For this review, take the finished solid that the model builds, in its own axes (mm). A direction names the side the tool comes from. Coordinates: 2 decimals unless noted, no trailing zeros. Write each loop counter-clockwise with the first axis right and the second up, starting at its lowest first coordinate (ties: lowest second). Pieces come first, ordered by that corner, then holes.
1) We need section D-D on y = 15.8. Write out the cut boundary in (x, z).
2) For faces 4 (the face through (28, 16, 0)), 5 (the face through (36, -35.8, -48)), 6 (the face through (26, 12, 0)), list the 3-axis set-ups (+Z, -Z, +X, -X, +Y, -Y) from which the entire face can be reached by the end or side of a thin tool; tool diameter is ignored.
3) We need section A-A on x = 30. Write out the cut boundary in (y, z).
4) To check wall thickness, follow line 1 along Y through (x, z) = (22, 0); line 2 along X through (y, z) = (-30.75, -64); line 3 along Y through (x, z) = (23.5, 0.5). State the ranges of each line that lie inside material, in increasing order.
5) Mouldability with a two-part tool opening along Y and no side actions: class faces 1 (the face through (34, -12, 28)), 2 (the face through (28.1, -39.7, -0.4)), 3 (the face through (36, -19.8, -48)) as pulls with the +Y half, pulls with the -Y half, needs draft (parallel to the pull), parting line crosses it, or undercut.
6) Insertion check: P1, Ø4.5, axis at y = -24.2, z = -16, coming from the -X side; P2, Ø8, axis at x = 31, z = -39.5, coming from the -Y side; P3, Ø2, axis at y = -33, z = -56.5, coming from the -X side. Each pin has a flat end and moves straight along its axis. Give the tip position at first contact, or say it passes through.
Autodesk Inventor part; units mm, degrees
ref_plane "YZ Plane" through (0, 0, 0) normal (1, 0, 0) x (0, 1, 0)
ref_plane "XZ Plane" through (0, 0, 0) normal (0, 1, 0) x (-1, 0, 0)
ref_plane "XY Plane" through (0, 0, 0) normal (0, 0, 1) x (1, 0, 0)
sketch "Sketch1" plane through (0, 0, 0) normal (1, 0, 0) x (0, 1, 0)
  line L0 (-19.8, 28) -> (19.8, 28)
  line L1 (19.8, 28) -> (19.8, -28)
  line L2 (19.8, -28) -> (-19.8, -28)
  line L3 (-19.8, -28) -> (-19.8, 28)
  line L4 (-19.8, 28) -> (19.8, -28) construction
  line L5 (19.8, 28) -> (-19.8, -28) construction
  point P0 (0, 0)
  dimension "d0" = 39.6
  dimension "d1" = 56
extrude "Extrusion1" add sketch "Sketch1" along normal blind 40
sketch "Sketch2" plane through (0, -19.8, 28) normal (0, 0, 1) x (1, 0, 0)
  line L0 (7.8, 0) -> (32.2, 0)
  line L1 (32.2, 0) -> (32.2, 31.8)
  line L2 (32.2, 31.8) -> (7.8, 31.8)
  line L3 (7.8, 31.8) -> (7.8, 0)
  line L4 (0, 0) -> (40, 0)
  line L5 (40, 39.6) -> (40, 0)
  dimension "d4" = 24.4
  dimension "d5" = 31.8
  dimension "d6" = 7.8
extrude "Extrusion2" cut sketch "Sketch2" against normal blind 64
sketch "Sketch3" plane through (32.2, -19.8, 28) normal (-1, 0, 0) x (0, 0, 1)
  circle A0 centre (-12, 3.8502) radius 2.3
  circle A1 centre (-28, 3.8502) radius 2.3
  line L0 (0, 31.8) -> (0, 0)
  point P0 (-28, 19.8)
  dimension "d9" = 4.6
  dimension "d10" = 4.6
  dimension "d11" = 16
  dimension "d12" = 12
extrude "Extrusion3" add sketch "Sketch3" along normal blind 26
sketch "Sketch4" plane through (7.8, -19.8, 28) normal (1, 0, 0) x (0, 0, -1)
  line L0 (56, 0) -> (0, 0)
  line L1 (56, 0) -> (32, 0)
  line L2 (32, 0) -> (32, 8)
  line L3 (32, 8) -> (56, 8)
  line L4 (56, 8) -> (56, 0)
  point P0 (28, 19.8)
  point P1 (32, 0)
  dimension "d15" = 24
  dimension "d16" = 8
extrude "Extrusion4" add sketch "Sketch4" along normal blind 26
sketch "Sketch14" plane through (0, 19.8, 28) normal (0, 1, 0) x (1, 0, 0)
  line L0 (20, 0) -> (20, 56)
  point P0 (0, 28)
sketch "Sketch15" plane through (0, -19.8, -28) normal (0, -1, 0) x (1, 0, 0)
  line L0 (40, 0) -> (40, 56)
  line L1 (0, 0) -> (40, 0)
  line L2 (0, 56) -> (40, 56)
  line L3 (0, 0) -> (0, 56)
  point P0 (0, 28)
extrude "Extrusion7" add sketch "Sketch15" along normal blind 24
sketch "Sketch16" plane through (0, 19.8, 28) normal (0, 0, 1) x (1, 0, 0)
  line L0 (8, -47.6) -> (32, -47.6)
  line L1 (32, -47.6) -> (32, -55.6)
  line L2 (32, -55.6) -> (8, -55.6)
  line L3 (8, -55.6) -> (8, -47.6)
  line L4 (40, -63.6) -> (0, -63.6)
  line L5 (0, 0) -> (0, -63.6)
  line L6 (16, -55.6) -> (24, -55.6)
  line L7 (24, -55.6) -> (24, -63.6)
  line L8 (24, -63.6) -> (16, -63.6)
  line L9 (16, -63.6) -> (16, -55.6)
  point P0 (0, -19.8)
  dimension "d37" = 24
  dimension "d38" = 8
  dimension "d39" = 8
  dimension "d40" = 8
  dimension "d41" = 8
  dimension "d42" = 8
  dimension "d43" = 16
extrude "Extrusion8" cut sketch "Sketch16" against normal through all
chamfer "Chamfer1" distance 8 angle 45 2 edges at (40, -43.8, 0) (0, -43.8, 0)
chamfer "Chamfer2" distance 8 angle 45 2 edges at (16, -35.8, 0) (24, -35.8, 0)
split body "Split2" sketch "Sketch14" result one side removed curves L0 removed pieces at (0.5, -17.2667, 9.3333)
sketch "Sketch17" plane through (20, -27.8, -28) normal (-1, 0, 0) x (0, 0, 1)
  circle A0 centre (12, 3.6) radius 2.5
  circle A1 centre (28, 3.6) radius 2.5
  circle A2 centre (44, 3.6) radius 2.5
  circle A3 centre (12, 43.6) radius 2.5
  circle A4 centre (44, 43.6) radius 2.5
  circle A5 centre (28, 43.6) radius 2.5
  line L0 (0, 47.6) -> (56, 47.6)
  line L1 (0, 39.8) -> (0, 47.6)
  point P0 (28, 27.8)
  dimension "d52" = 5
  dimension "d53" = 5
  dimension "d55" = 5
  dimension "d56" = 5
  dimension "d57" = 5
  dimension "d58" = 5
  dimension "d59" = 16
  dimension "d60" = 16
  dimension "d61" = 40
  dimension "d62" = 4
  dimension "d63" = 12
extrude "Extrusion9" cut sketch "Sketch17" against normal blind 8
sketch "Sketch22" plane through (32.2, -11.8, -28) normal (0, 0, -1) x (-1, 0, 0)
  line L0 (0.2, -32) -> (-7.8, -24)
  line L1 (-7.8, -24) -> (0.2, -24)
  line L2 (0.2, -24) -> (0.2, -8)
  line L3 (0.2, -8) -> (-7.8, -8)
  line L4 (-7.8, -8) -> (-7.8, -24)
  point P0 (32.2, 11.8)
  dimension "d82" = 8
  dimension "d83" = 16
extrude "Extrusion13" add sketch "Sketch22" along normal blind 39.7
sketch "Sketch23" plane through (32, -19.8, -28) normal (0, 1, 0) x (1, 0, 0)
  circle A0 centre (4, 36) radius 2.5
  line L0 (8, 0) -> (8, 39.7)
  line L1 (0, 39.7) -> (8, 39.7)
  point P0 (-32, -28)
  dimension "d86" = 5
  dimension "d87" = 4
  dimension "d88" = 3.7
extrude "Extrusion14" cut sketch "Sketch23" against normal through all
fillet "Fillet2" radius 4 2 edges at (40, -27.8, -67.7) (32, -27.8, -67.7)
properties part number "MotorHolder_X_R"
Result:
1. outline: (20, -28) - (40, -28) - (40, 28) - (20, 28) - (20, 18.5) - (28, 18.5) - (28, 13.5) - (20, 13.5) - (20, 2.5) - (28, 2.5) - (28, -2.5) - (20, -2.5) - (20, -13.5) - (28, -13.5) - (28, -18.5) - (20, -18.5) - close
2. face 4: -X
2. face 5: -Z, +X, -X, -Y
2. face 6: +Z, -Z, -X
3. outline: (-43.8, -28) - (-37.8, -28) - (-37.8, 28) - (-43.8, 28) - close; (-27.8, -28) - (-11.8, -28) - (-11.8, -4) - (-19.8, -4) - (-19.8, 28) - (-27.8, 28) - close; circle Ø4.6 at (-15.95, 0); circle Ø4.6 at (-15.95, 16); (12, -28) - (19.8, -28) - (19.8, 28) - (12, 28) - close
4. line 1: y = -27.8 to -26.7, -21.7 to -19.8, -18.25 to -13.65, 12 to 13.3, 18.3 to 19.8
4. line 2: x = 32.01 to 33.5, 38.5 to 39.99
4. line 3: y = -27.8 to -26.65, -21.75 to -19.8, -18.19 to -13.7, 12 to 13.35, 18.25 to 19.8
5. face 1: needs draft
5. face 2: undercut
5. face 3: pulls with the +Y half
6. P1: stops at x = 28
6. P2: stops at y = -35.8
6. P3: stops at x = 32
